Design review of the part built by this model. Coordinates are the model's own, in mm. Coordinates: 2 decimals unless noted, no trailing zeros. Loops run counter-clockwise (first coordinate to the right, second up) from the corner with the lowest first, then second, coordinate; pieces in that order, holes last. Notation, with made-up numbers: (58, -12) - (90, -12) arc R33 ccw to (90, 22) - close; hole circle Ø5 at (32, -32). An arc over 180 degrees is marked (long way). One line per question, with ' | ' between items.
from build123d import *

# Parameters (mm, degrees)
F0_W     = 25.4
F0_H     = 25.4
F0_W_2   = 22.225
F0_H_2   = 22.225
F1_DEPTH = 304.8
F2_R     = 4.7625
F3_DEPTH = 25.4


with BuildPart() as f1:
    # F0 (on Right) → F1 (new body)
    with BuildSketch(Plane.YZ):
        with Locations((-11.1125, -9.054881)):
            Rectangle(F0_W, F0_H)
        with Locations((-11.1125, -9.054881)):
            Rectangle(F0_W_2, F0_H_2, mode=Mode.SUBTRACT)
    extrude(amount=F1_DEPTH)

    # F2 (on face) → F3 (cut)
    with BuildSketch(Plane.XZ.offset(23.8125)):
        with Locations((25.4, -9.054881)):
            Circle(F2_R)
    extrude(amount=-F3_DEPTH, mode=Mode.SUBTRACT)


solid = f1.part
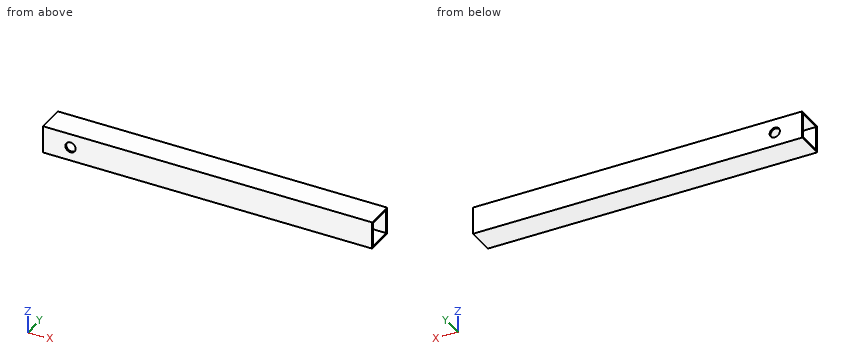
Q1. Take a section at A-A (y = -14.25). Give the boundary of the cut face in (x, z), plus the area to 3 significant figures.
Returned:
outline: (0, -21.75) - (304.8, -21.75) - (304.8, -20.17) - (0, -20.17) - close; (0, 2.06) - (304.8, 2.06) - (304.8, 3.65) - (0, 3.65) - close | area: 968 mm²
Q2. Take a section at C-C (z = -1). Give the boundary of the cut face in (x, y) (1 decimal).
Returned:
outline: (0, -23.8) - (304.8, -23.8) - (304.8, -22.2) - (0, -22.2) - close; (0, 0) - (304.8, 0) - (304.8, 1.6) - (0, 1.6) - close
Q3. Take a section at D-D (x = 254.5). Give the boundary of the cut face in (y, z) (1 decimal).
Returned:
outline: (-23.8, -21.8) - (1.6, -21.8) - (1.6, 3.6) - (-23.8, 3.6) - close; hole (-22.2, -20.2) - (0, -20.2) - (0, 2.1) - (-22.2, 2.1) - close
Q4. Take a section at B-B (x = 25.4). Give the boundary of the cut face in (y, z) (1 decimal).
Returned:
outline: (-23.8, -21.8) - (1.6, -21.8) - (1.6, -13.8) - (0, -13.8) - (0, -20.2) - (-22.2, -20.2) - (-22.2, -13.8) - (-23.8, -13.8) - close; (-23.8, -4.3) - (-22.2, -4.3) - (-22.2, 2.1) - (0, 2.1) - (0, -4.3) - (1.6, -4.3) - (1.6, 3.6) - (-23.8, 3.6) - close
Q5. For pin 1 (10 mm diameter, centred on y = -18.5, z = -8.5, fed in from -X), flat-tipped, find the tip position at first contact; note if it passes through.
Returned:
pin 1: stops at x = 0
Q6. To check wall thickness, follow line 1 along Y through (x, z) = (213, -7.5) (1 decimal); line 2 along Z through (x, y) = (66.5, -8); line 3 along Z through (x, y) = (25.4, -22.8). State the ranges of each line that lie inside material, in increasing order.
Returned:
line 1: y = -23.8 to -22.2, 0 to 1.6 | line 2: z = -21.75 to -20.17, 2.06 to 3.65 | line 3: z = -21.75 to -13.82, -4.29 to 3.65
